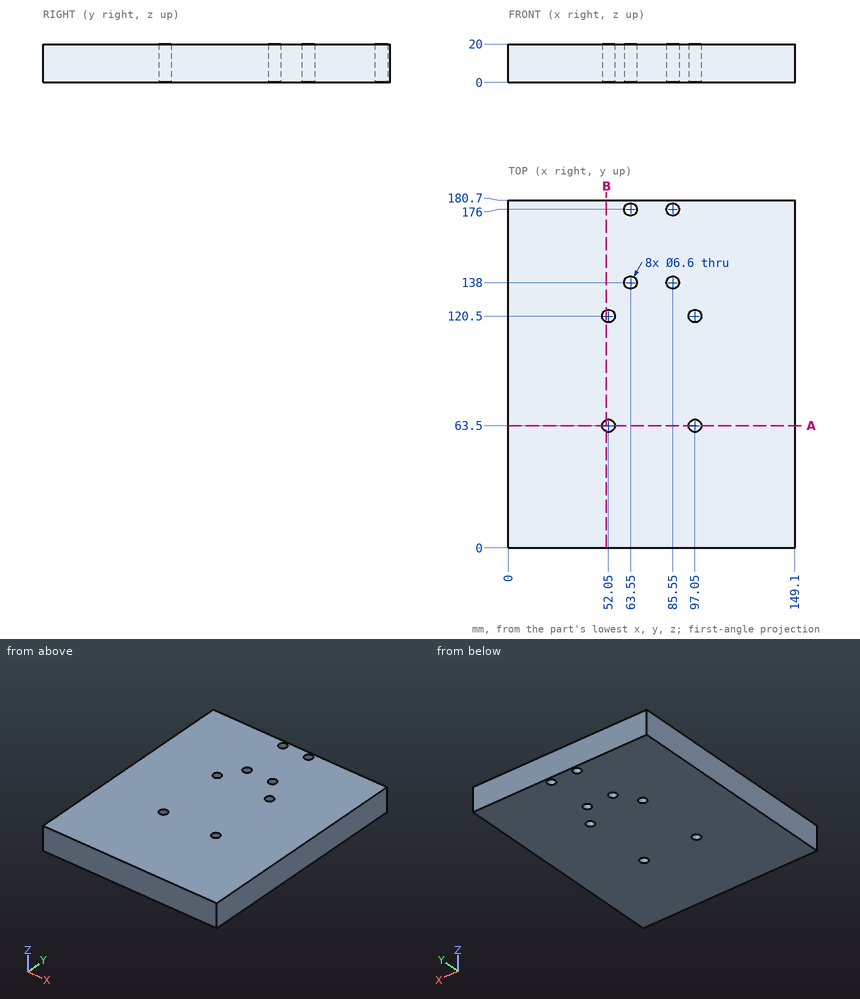
Study the drawing (mm; zero at the part's minimum x, y, z) and answer. Give positions to 0.01 mm unless a question says otherwise; leave off trailing zeros. Write each loop counter-clockwise with the first axis right and the second up, starting at its lowest first coordinate (ties: lowest second). Pieces come first, ordered by that corner, then holes.
Item 1: Section B-B, the plane x = 51 is taken. Write down the section's boundary in (y, z), plus the area to 3 significant figures.
Item 2: A flat-ended cylindrical pin translates along its axis: P1, Ø2, axis at y = 74.5, z = 10, coming from the -X side. Find the tip coordinate at first contact, or state that the pin passes through.
Item 3: Find the intervals of material crossed by line 1 along Y through (x, z) = (85.5, 4.25); line 2 along X through (y, z) = (176, 4.75); line 3 along Y through (x, z) = (100, 7.25) (1 decimal), in increasing order.
Item 4: Section A-A, the plane y = 63.5 is taken. Write down the section's boundary in (x, z), plus the area to 3 significant figures.
Completed:
1. outline: (0, 0) - (60.37, 0) - (60.37, 20) - (0, 20) - close; (66.63, 0) - (117.37, 0) - (117.37, 20) - (66.63, 20) - close; (123.63, 0) - (180.7, 0) - (180.7, 20) - (123.63, 20) - close
1. area: 3,360 mm2
2. P1: stops at x = 0
3. line 1: y = 0 to 134.7, 141.3 to 172.7, 179.3 to 180.7
3. line 2: x = 0 to 60.25, 66.85 to 82.25, 88.85 to 149.1
3. line 3: y = 0 to 62, 65 to 119, 122 to 180.7
4. outline: (0, 0) - (48.75, 0) - (48.75, 20) - (0, 20) - close; (55.35, 0) - (93.75, 0) - (93.75, 20) - (55.35, 20) - close; (100.35, 0) - (149.1, 0) - (149.1, 20) - (100.35, 20) - close
4. area: 2,720 mm2
